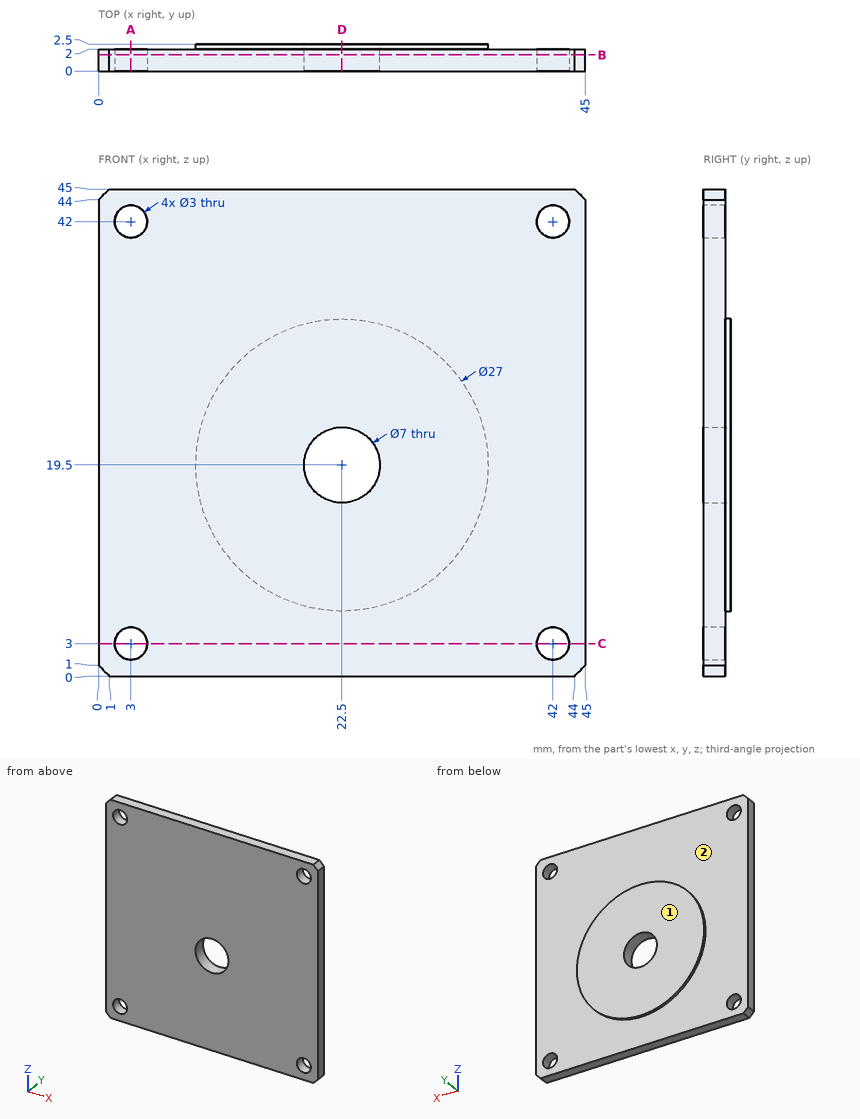
Check sheet for the drawn part. Datum: minimum x, y, z corner. Units: mm. A direction names the side the tool comes from. Coordinates: 2 decimals unless noted, no trailing zeros. Order: outer loops, then holes, each group sorted by start corner. A loop starts at its lowest first (then second) coordinate and runs counter-clockwise, first axis right, second up. Notation, with made-up numbers: M 24.5,78.25 L 69.5,78.25 A19 ccw 69.5,89.25 Z; hole C 76.5,75 d6. An arc over 180 degrees is marked long. One line per item, written item: value. Start each with the question number.
Item 1: Gauge pin test, flat end, axial feed: pin 1 (5 mm diameter, centred on x = 42, z = 3, fed in from -Y). Record the tip position at first contact, or that the pin passes through.
Item 2: Sectioned sample at A-A (x = 3). Enter the section's corners in (y, z), then the cut area to 3 significant figures.
Item 3: Sectioned sample at D-D (x = 22.5). Enter the section's corners in (y, z).
Item 4: Sectioned sample at C-C (z = 3). Enter the section's corners in (x, y).
Item 5: Sectioned sample at B-B (y = 1.5). Enter the section's corners in (x, z), then the cut area to 3 significant figures.
Item 6: Access from +Z, -Z, +X, -X, +Y, -Y to the whole of each face (thin tool, end or side, straight path). Record for the marked faces 1 and 2.
Item 7: Scan lines: probe 1 along X at (y, z) = (0.75, 3); probe 2 along X at (y, z) = (0.85, 4). Record each from-to range of solid material in increasing order.
Conclusion:
1. pin 1: stops at y = 0
2. outline: M 0,0 L 2,0 L 2,1.5 L 0,1.5 Z; M 0,4.5 L 2,4.5 L 2,40.5 L 0,40.5 Z; M 0,43.5 L 2,43.5 L 2,45 L 0,45 Z
2. area: 78.0 mm^2
3. outline: M 0,0 L 2,0 L 2,6 L 2.5,6 L 2.5,16 L 0,16 Z; M 0,23 L 2.5,23 L 2.5,33 L 2,33 L 2,45 L 0,45 Z
4. outline: M 0,0 L 1.5,0 L 1.5,2 L 0,2 Z; M 4.5,0 L 40.5,0 L 40.5,2 L 4.5,2 Z; M 43.5,0 L 45,0 L 45,2 L 43.5,2 Z
5. outline: M 0,1 L 1,0 L 44,0 L 45,1 L 45,44 L 44,45 L 1,45 L 0,44 Z; hole C 3,3 d3; hole C 3,42 d3; hole C 22.5,19.5 d7; hole C 42,3 d3; hole C 42,42 d3
5. area: 1,960 mm^2
6. face 1: +Z, -Z, +X, -X, +Y
6. face 2: +Y
7. probe 1: x = 0 to 1.5, 4.5 to 40.5, 43.5 to 45
7. probe 2: x = 0 to 1.88, 4.12 to 40.88, 43.12 to 45
